Input: part model. Units: mm. Frame: model coordinates. Round coordinates to 2 decimals unless told otherwise and drop trailing zeros. Loops run counter-clockwise (first coordinate to the right, second up) from the corner with the lowest first, then second, coordinate; pieces in that order, holes last. Notation, with made-up numbers: (38, 36.5) -> (49, 36.5) arc R14 cw to (49, 42.5) -> close; hole circle Ø3 at (-21.5, 50). An arc over 180 degrees is marked (long way). Answer in a Markdown table with one row per item. Add a question column.
Q1. Ray query, L1, parallel to Z at x = 0, y = -36; L2, parallel to Z at x = -6.5, y = -41; L3, parallel to X at y = -45, z = 3.5. Return the intervals inside material, ascending. Write a range as from..to.
Q2. Section C-C, the plane y = -16. Output: boundary loops of the cut face in (x, z).
Q3. Section A-A, the plane z = 0. Output: boundary loops of the cut face in (x, y).
Q4. Section B-B, the plane x = 0. Output: boundary loops of the cut face in (y, z).
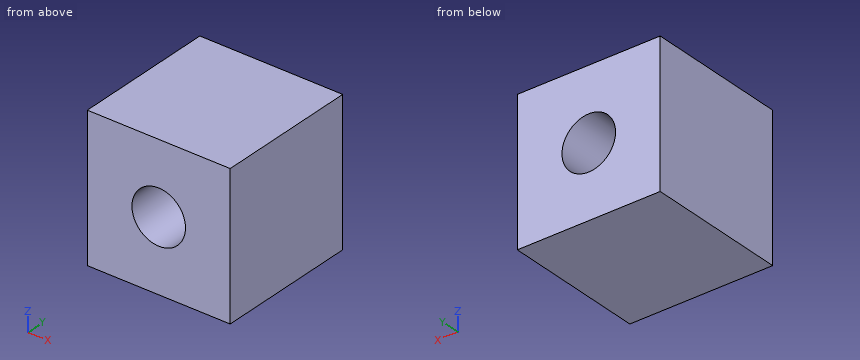
```python
from build123d import *

# Parameters (mm, degrees)
F0_W     = 48
F0_H     = 48
F1_DEPTH = 48
F3_D     = 18


with BuildPart() as f1:
    # F0 (on Front) → F1 (new body)
    with BuildSketch(Plane.XZ):
        Rectangle(F0_W, F0_H)
    extrude(amount=F1_DEPTH)

    # F3 (through all)
    with Locations(Plane(origin=(0, 0, 0), x_dir=(1, 0, 0), z_dir=(0, 1, 0))):
        with Locations((0, 0)):
            Hole(F3_D / 2)


solid = f1.part
```
Answer block:
| question | item | result |
|---|---|---|
| 1 | L1 | -24..-9, 9..24 |
| 1 | L2 | -24..-6.22, 6.22..24 |
| 1 | L3 | -24..-8.29, 8.29..24 |
| 2 | outline | (-24, -24) -> (24, -24) -> (24, 24) -> (-24, 24) -> close; hole circle Ø18 at (0, 0) |
| 3 | outline | (-24, -48) -> (-9, -48) -> (-9, 0) -> (-24, 0) -> close; (9, -48) -> (24, -48) -> (24, 0) -> (9, 0) -> close |
| 4 | outline | (-48, -24) -> (0, -24) -> (0, -9) -> (-48, -9) -> close; (-48, 9) -> (0, 9) -> (0, 24) -> (-48, 24) -> close |
